Geometry: final body of the model. Coordinates: model frame, mm. Give positions to 0.01 mm unless a question says otherwise; leave off trailing zeros. Order: outer loops, then holes, each group sorted by start corner. A loop starts at its lowest first (then second) coordinate and runs counter-clockwise, first axis right, second up. Notation, with made-up numbers: (-40, 58.5) -> (4, 58.5) arc R28 cw to (4, 97.5) -> close; hole circle Ø7 at (76, -2.75). An arc over 180 degrees is marked (long way). One line per question, with ' | ' between items.
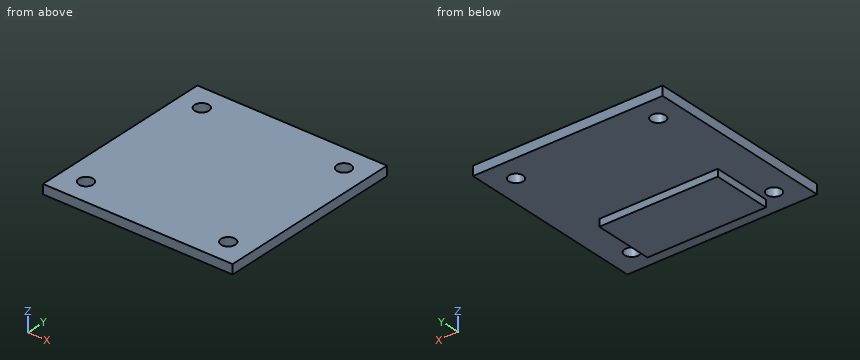
from build123d import *

# Parameters (mm, degrees)
F0_W     = 80
F0_H     = 80
F1_DEPTH = 4
F2_W     = 50
F2_H     = 25
F3_DEPTH = 3
F4_D     = 6


with BuildPart() as f1:
    # F0 (on Top) → F1 (new body)
    with BuildSketch(Plane.XY):
        Rectangle(F0_W, F0_H)
    extrude(amount=F1_DEPTH)

    # F2 (on face) → F3 (join)
    with BuildSketch(Plane(origin=(0, 0, 0), x_dir=(1, 0, 0), z_dir=(0, 0, -1))):
        with Locations((0, 19.5)):
            Rectangle(F2_W, F2_H)
    extrude(amount=F3_DEPTH)

    # F4 (through all)
    with Locations(Plane(origin=(0, 0, 0), x_dir=(1, 0, 0), z_dir=(0, 0, -1))):
        with Locations((-30, 30), (30, 30), (30, -30), (-30, -30)):
            Hole(F4_D / 2)


solid = f1.part
1) Contact query for flat-ended pins moving along their axis: pin 1 Ø3.5 at (x, z) = (0, -2) entering from +Y; pin 2 Ø0.9 at (x, z) = (-7.5, -1.5) entering from -Y; pin 3 Ø10 at (x, y) = (-29, 14) entering from -Z. Output: stop coordinate, or through.
Check result:
pin 1: stops at y = -7 | pin 2: stops at y = -32 | pin 3: stops at z = 0
2) Section D-D on x = -9.5. Return loops of the section in (y, z), plus the area to 3 significant figures.
Check result:
outline: (-40, 0) -> (-32, 0) -> (-32, -3) -> (-7, -3) -> (-7, 0) -> (40, 0) -> (40, 4) -> (-40, 4) -> close | area: 395 mm^2
3) Material intervals for probe 1 along Y at (x, z) = (30, 1.55); probe 2 along Z at (x, y) = (9.5, 1), sorted ascending. Write a range as from..to.
Check result:
probe 1: y = -40..-33, -27..27, 33..40 | probe 2: z = 0..4
4) Section C-C on z = 2. Return loops of the section in (x, y).
Check result:
outline: (-40, -40) -> (40, -40) -> (40, 40) -> (-40, 40) -> close; hole circle Ø6 at (-30, -30); hole circle Ø6 at (-30, 30); hole circle Ø6 at (30, -30); hole circle Ø6 at (30, 30)
5) Section A-A on y = 30. Return loops of the section in (x, z), plus the area to 3 significant figures.
Check result:
outline: (-40, 0) -> (-33, 0) -> (-33, 4) -> (-40, 4) -> close; (-27, 0) -> (27, 0) -> (27, 4) -> (-27, 4) -> close; (33, 0) -> (40, 0) -> (40, 4) -> (33, 4) -> close | area: 272 mm^2
